Could you check a few things on this model? Use its own coordinates, in mm. Face numbers are marked on the shaded views. Give positions to 0.01 mm unless a question says otherwise; leave off trailing zeros. Write each loop counter-clockwise with the first axis right and the second up, starting at its lowest first coordinate (ties: lowest second). Pieces come first, ordered by that corner, then holes. Notation, with made-up numbers: M 36.25,19.5 L 63.25,19.5 A21 ccw 63.25,27.5 Z; hole C -13,58.5 d2. An arc over 180 degrees is marked long. Use one line per item in the form item = value.
from build123d import *

# Parameters (mm, degrees)
SCHIZZO3_R               = 1.5
TAGLIO_ESTRUSIONE1_DEPTH = 6
SMUSSO1_SIZE             = 0.5


with BuildPart() as part:
    # Schizzo1 → Rivoluzione1 (revolve)
    with BuildSketch(Plane.XY):
        with BuildLine():
            Line((0, 5), (0, -5))
            ThreePointArc((0, -5), (-5, 0), (0, 5))
        make_face()
    revolve(axis=Axis((0, 5, 0), (0, -1, 0)))

    # Schizzo2 → Taglia-Rivoluzione1 (revolve, cut)
    with BuildSketch(Plane.XY, mode=Mode.PRIVATE) as taglia_rivoluzione1_sk:
        with BuildLine():
            Line((0, 3.5), (-3.570714214, 3.5))
            ThreePointArc((-3.570714214, 3.5), (-1.936491673, 4.609772229), (0, 5))
            Line((0, 5), (0, 3.5))
        make_face()
    revolve(taglia_rivoluzione1_sk.sketch.rotate(Axis((0, 5, 0), (0, -1, 0)), 180), axis=Axis((0, 5, 0), (0, -1, 0)), mode=Mode.SUBTRACT)

    # Schizzo3 → Taglio-Estrusione1 (cut)
    with BuildSketch(Plane(origin=(0, 3.5, 0), x_dir=(1, 0, 0), z_dir=(0, 1, 0))):
        with Locations(Location((0, 0, 0), (0, 0, 270))):
            Circle(SCHIZZO3_R)
    extrude(amount=-TAGLIO_ESTRUSIONE1_DEPTH, mode=Mode.SUBTRACT)

    # Smusso1
    smusso1_edges = [part.edges().sort_by_distance(p)[0] for p in [
        (0, 3.5, -1.5),
    ]]
    chamfer(smusso1_edges, length=SMUSSO1_SIZE)


solid = part.part
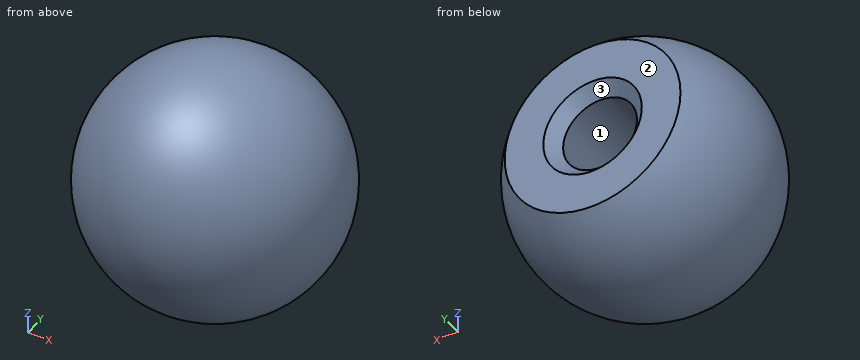
1) For pin 1 Ø1 at (x, y) = (-2, 1) entering from +Z; pin 2 Ø0.9 at (x, z) = (0.5, -0.5) entering from +Y; pin 3 Ø2 at (x, z) = (-3, 3.5) entering from -Y, each with a flat end and sliding along its axis, tell me the tip position at first contact or that it passes through.
Checked values:
pin_1 = 4.69
pin_2 = -2.5
pin_3 = -3.46
2) If I drill on L1, parallel to Z at x = 1.25, y = -1.75; L2, parallel to X at y = 0.7, z = 0; L3, parallel to Z at x = -0.25, y = -2.25, over which ranges is the centre line in solid material (lowest first)?
Checked values:
L1 = -4.51 to -0.83, 0.83 to 4.51
L2 = -4.95 to -1.5, 1.5 to 4.95
L3 = -4.46 to -1.48, 1.48 to 4.46
3) I want a section at C-C, the plane y = -4. Please give me the cut outline in (x, z).
Checked values:
outline = C 0,0 d6
4) Thinking about a two-plate mould opening in X: for the marked faces 1, 2 and 3, which applies, released by +X, released by -X, zero draft, split by the parting line, or undercut?
Checked values:
face_1 = undercut
face_2 = zero draft
face_3 = undercut
5) I want a section at B-B, the plane x = 0. Please give me the cut outline in (y, z).
Checked values:
outline = M -2.5,-1.5 L -2.5,1.5 L 3,1.5 L 3.5,2 L 3.5,3.57 A5 ccw long 3.5,-3.57 L 3.5,-2 L 3,-1.5 Z
6) I want a section at D-D, the plane y = -0.25. Please give me the cut outline in (x, z).
Checked values:
outline = C 0,0 d9.99; hole C 0,0 d3
7) I want a section at A-A, the plane z = 0. Please give me the cut outline in (x, y).
Checked values:
outline = M -3.57,3.5 A5 ccw long 3.57,3.5 L 2,3.5 L 1.5,3 L 1.5,-2.5 L -1.5,-2.5 L -1.5,3 L -2,3.5 Z
